from build123d import *

# Parameters (mm, degrees)
SKETCH1_W                     = 190.5
SKETCH1_H                     = 101.6
BOSS_EXTRUDE1_DEPTH           = 1.5875
CONVERT_SOLID1_START          = -95.25
CONVERT_SOLID1_OUTLINE_W      = 3.175
CONVERT_SOLID1_OUTLINE_H      = 101.6
CONVERT_SOLID1_DEPTH          = 190.5
SKETCH30_R                    = 12.770921212
CUT_EXTRUDE6_DEPTH            = 38.1
SKETCH35_W                    = 139.601875342
SKETCH35_H                    = 6.35
CUT_EXTRUDE7_DEPTH            = 0.254
EDGE_FLANGE1_STRIP_W          = 39.05
EDGE_FLANGE1_STRIP_H          = 4.7625
EDGE_FLANGE1_STRIP_CUT_DEPTH  = 25.449062329
EDGE_FLANGE1_RELIEF_W         = 41.43125
EDGE_FLANGE1_RELIEF_H         = 2.38125
EDGE_FLANGE1_RELIEF_CUT_DEPTH = 4.7625
EDGE_FLANGE1_DEPTH            = 25.449062329
EDGE_FLANGE2_STRIP_W          = 39.05
EDGE_FLANGE2_STRIP_H          = 4.7625
EDGE_FLANGE2_STRIP_CUT_DEPTH  = 25.449062329
EDGE_FLANGE2_RELIEF_W         = 41.43125
EDGE_FLANGE2_RELIEF_H         = 2.38125
EDGE_FLANGE2_RELIEF_CUT_DEPTH = 4.7625
EDGE_FLANGE2_DEPTH            = 25.449062329
SKETCH45_W                    = 4.7625
SKETCH45_H                    = 0.000254
CUT_EXTRUDE10_DEPTH           = 25.4
EDGE_FLANGE4_STRIP_W          = 39.05
EDGE_FLANGE4_STRIP_H          = 4.7625
EDGE_FLANGE4_STRIP_CUT_DEPTH  = 25.4
EDGE_FLANGE4_RELIEF_W         = 41.43125
EDGE_FLANGE4_RELIEF_H         = 2.38125
EDGE_FLANGE4_RELIEF_CUT_DEPTH = 4.7625
EDGE_FLANGE4_DEPTH            = 25.4
FILLET9_R                     = 25.4
CUT_EXTRUDE11_DEPTH           = 25.4
FILLET10_R                    = 25.4
SKETCH53_R                    = 2.54
CUT_EXTRUDE12_DEPTH           = 4.7625
SKETCH54_R                    = 2.54
CUT_EXTRUDE13_DEPTH           = 4.7625
SKETCH55_R                    = 9.525
SKETCH55_R_2                  = 2.54
CUT_EXTRUDE14_DEPTH           = 4.7625


# Read off the part's stored shape, not the designer's step: Convert-Solid1
# Sheet-metal steps are written as plain solids
with BuildPart() as part:
    # Sketch1 → Boss-Extrude1 (new body)
    with BuildSketch(Plane(origin=(0, 0, 0), x_dir=(1, 0, 0), z_dir=(0, 1, 0))):
        Rectangle(SKETCH1_W, SKETCH1_H)
    extrude(amount=BOSS_EXTRUDE1_DEPTH)

    # Convert-Solid1 outline → Convert-Solid1 (add)
    with BuildSketch(Plane.YZ.offset(CONVERT_SOLID1_START)):
        with Locations((-1.5875, 0)):
            Rectangle(CONVERT_SOLID1_OUTLINE_W, CONVERT_SOLID1_OUTLINE_H)
    extrude(amount=CONVERT_SOLID1_DEPTH)

    # Sketch30 → Cut-Extrude6 (cut)
    with BuildSketch(Plane(origin=(0, -3.175, 0), x_dir=(-1, 0, 0), z_dir=(0, -1, 0))):
        with Locations(Location((0, -25.504506424, 0), (0, 0, 90))):
            Circle(SKETCH30_R)
    extrude(amount=-CUT_EXTRUDE6_DEPTH, mode=Mode.SUBTRACT)

    # Sketch35 → Cut-Extrude7 (cut)
    with BuildSketch(Plane(origin=(0, 0, -50.8), x_dir=(-1, 0, 0), z_dir=(0, 0, -1))):
        Rectangle(SKETCH35_W, SKETCH35_H)
    extrude(amount=-CUT_EXTRUDE7_DEPTH, mode=Mode.SUBTRACT)

    # Edge-Flange1 strip (across the edge) → Edge-Flange1 strip cut (cut)
    with BuildSketch(Plane(origin=(95.25, 1.5875, -50.8), x_dir=(0, 0, 1), z_dir=(-1, 0, 0))):
        with Locations((-4.7625, -2.38125)):
            Rectangle(EDGE_FLANGE1_STRIP_W, EDGE_FLANGE1_STRIP_H)
    extrude(amount=EDGE_FLANGE1_STRIP_CUT_DEPTH, mode=Mode.SUBTRACT)

    # Edge-Flange1 relief (on the sheet) → Edge-Flange1 relief cut (cut)
    with BuildSketch(Plane(origin=(95.25, 1.5875, -36.0375), x_dir=(0, 0, 1), z_dir=(0, 1, 0))):
        with Locations((-18.334375, -26.639687329)):
            Rectangle(EDGE_FLANGE1_RELIEF_W, EDGE_FLANGE1_RELIEF_H)
    extrude(amount=-EDGE_FLANGE1_RELIEF_CUT_DEPTH, mode=Mode.SUBTRACT)

    # Edge-Flange1 section (across the edge) → Edge-Flange1 (add)
    with BuildSketch(Plane(origin=(95.25, 1.5875, -50.8), x_dir=(0, 0, 1), z_dir=(-1, 0, 0))):
        with BuildLine():
            Line((0, 10), (0, 46.0375))
            Line((0, 46.0375), (4.7625, 46.0375))
            Line((4.7625, 46.0375), (4.7625, 10))
            ThreePointArc((4.7625, 10), (7.691432188, 2.928932188), (14.7625, 0))
            Line((14.7625, 0), (14.7625, -4.7625))
            ThreePointArc((14.7625, -4.7625), (4.323836143, -0.438663857), (0, 10))
        make_face()
    extrude(amount=EDGE_FLANGE1_DEPTH)

    # Edge-Flange2 strip (across the edge) → Edge-Flange2 strip cut (cut)
    with BuildSketch(Plane(origin=(-69.800937671, 1.5875, -50.8), x_dir=(0, 0, 1), z_dir=(-1, 0, 0))):
        with Locations((-4.7625, -2.38125)):
            Rectangle(EDGE_FLANGE2_STRIP_W, EDGE_FLANGE2_STRIP_H)
    extrude(amount=EDGE_FLANGE2_STRIP_CUT_DEPTH, mode=Mode.SUBTRACT)

    # Edge-Flange2 relief (on the sheet) → Edge-Flange2 relief cut (cut)
    with BuildSketch(Plane(origin=(-69.800937671, 1.5875, -36.0375), x_dir=(0, 0, 1), z_dir=(0, 1, 0))):
        with Locations((-18.334375, 1.190625)):
            Rectangle(EDGE_FLANGE2_RELIEF_W, EDGE_FLANGE2_RELIEF_H)
    extrude(amount=-EDGE_FLANGE2_RELIEF_CUT_DEPTH, mode=Mode.SUBTRACT)

    # Edge-Flange2 section (across the edge) → Edge-Flange2 (add)
    with BuildSketch(Plane(origin=(-69.800937671, 1.5875, -50.8), x_dir=(0, 0, 1), z_dir=(-1, 0, 0))):
        with BuildLine():
            Line((0, 10), (0, 46.0375))
            Line((0, 46.0375), (4.7625, 46.0375))
            Line((4.7625, 46.0375), (4.7625, 10))
            ThreePointArc((4.7625, 10), (7.691432188, 2.928932188), (14.7625, 0))
            Line((14.7625, 0), (14.7625, -4.7625))
            ThreePointArc((14.7625, -4.7625), (4.323836143, -0.438663857), (0, 10))
        make_face()
    extrude(amount=EDGE_FLANGE2_DEPTH)

    # Sketch45 → Cut-Extrude10 (cut)
    with BuildSketch(Plane(origin=(0, 1.5875, 0), x_dir=(1, 0, 0), z_dir=(0, 1, 0))):
        with Locations((-92.86875, -25.399873)):
            Rectangle(SKETCH45_W, SKETCH45_H)
        with Locations((-92.86875, 0.000381)):
            Rectangle(SKETCH45_W, SKETCH45_H)
    extrude(amount=-CUT_EXTRUDE10_DEPTH, mode=Mode.SUBTRACT)

    # Edge-Flange4 strip (across the edge) → Edge-Flange4 strip cut (cut)
    with BuildSketch(Plane(origin=(-95.25, 1.5875, -0.000254), x_dir=(1, 0, 0), z_dir=(0, 0, 1))):
        with Locations((-9.525, -2.38125)):
            Rectangle(EDGE_FLANGE4_STRIP_W, EDGE_FLANGE4_STRIP_H)
    extrude(amount=EDGE_FLANGE4_STRIP_CUT_DEPTH, mode=Mode.SUBTRACT)

    # Edge-Flange4 relief (on the sheet) → Edge-Flange4 relief cut (cut)
    with BuildSketch(Plane(origin=(-85.25, 1.5875, -0.000254), x_dir=(1, 0, 0), z_dir=(0, 1, 0))):
        with Locations((-18.334375, 1.190625)):
            Rectangle(EDGE_FLANGE4_RELIEF_W, EDGE_FLANGE4_RELIEF_H)
        with Locations((-18.334375, -26.590625)):
            Rectangle(EDGE_FLANGE4_RELIEF_W, EDGE_FLANGE4_RELIEF_H)
    extrude(amount=-EDGE_FLANGE4_RELIEF_CUT_DEPTH, mode=Mode.SUBTRACT)

    # Edge-Flange4 section (across the edge) → Edge-Flange4 (add)
    with BuildSketch(Plane(origin=(-95.25, 1.5875, -0.000254), x_dir=(1, 0, 0), z_dir=(0, 0, 1))):
        with BuildLine():
            Line((-4.7625, 10), (-4.7625, 20.6375))
            Line((-4.7625, 20.6375), (0, 20.6375))
            Line((0, 20.6375), (0, 10))
            ThreePointArc((0, 10), (2.928932188, 2.928932188), (10, 0))
            Line((10, 0), (10, -4.7625))
            ThreePointArc((10, -4.7625), (-0.438663857, -0.438663857), (-4.7625, 10))
        make_face()
    extrude(amount=EDGE_FLANGE4_DEPTH)

    # Fillet9
    # the kernel refuses this fillet: 25.4 mm, written as the material it takes off along each edge
    with BuildSketch(Plane(origin=(-67.419687671, 61.417239936, -50.546), x_dir=(1, 0, 0), z_dir=(0, -1, 0))) as fillet9_piece_1:
        with BuildLine():
            CenterArc((23.931895975, 25.4), FILLET9_R, 199.575530564, 70.424469436)
            Line((0, 16.88975), (-0.478637919, 16.719545))
            ThreePointArc((-0.478637919, 16.719545), (-0.508, 8.444875), (-0.508, 0))
            Line((-0.508, 0), (0, -0.508))
            Line((0, -0.508), (23.931895975, -0.508))
            Line((23.931895975, -0.508), (23.931895975, 0))
        make_face()
    extrude(amount=124.421979873, mode=Mode.SUBTRACT)
    with BuildSketch(Plane(origin=(67.419687671, 61.417239936, -50.546), x_dir=(0, 0, 1), z_dir=(0, -1, 0))) as fillet9_piece_2:
        with BuildLine():
            CenterArc((25.4, 23.931895975), FILLET9_R, 180, 70.424469436)
            Line((0, 23.931895975), (-0.508, 23.931895975))
            Line((-0.508, 23.931895975), (-0.508, 0))
            Line((-0.508, 0), (0, -0.508))
            ThreePointArc((0, -0.508), (8.444875, -0.508), (16.719545, -0.478637919))
            Line((16.719545, -0.478637919), (16.88975, 0))
        make_face()
    extrude(amount=124.421979873, mode=Mode.SUBTRACT)

    # Sketch52 → Cut-Extrude11 (cut)
    with BuildSketch(Plane.XZ.offset(3.175)):
        with BuildLine():
            ThreePointArc((62.156767956, 50.8), (84.936935051, 40.486935051), (95.25, 17.706767956))
            Line((95.25, 17.706767956), (95.25, 50.8))
            Line((95.25, 50.8), (62.156767956, 50.8))
        make_face()
    extrude(amount=-CUT_EXTRUDE11_DEPTH, mode=Mode.SUBTRACT)

    # Fillet10
    # the kernel refuses this fillet: 25.4 mm, written as the material it takes off along each edge
    with BuildSketch(Plane(origin=(-95.25, 64.807891195, 50.8), x_dir=(1, 0, 0), z_dir=(0, -1, 0))) as fillet10_piece_1:
        with BuildLine():
            CenterArc((25.288156478, -25.4), FILLET10_R, 90, 84.621196501)
            Line((0, -23.019004), (-0.50576313, -22.97138408))
            ThreePointArc((-0.50576313, -22.97138408), (-0.508, -11.509502), (-0.508, 0))
            Line((-0.508, 0), (0, 0.508))
            Line((0, 0.508), (25.288156478, 0.508))
            Line((25.288156478, 0.508), (25.288156478, 0))
        make_face()
    extrude(amount=131.203282389, mode=Mode.SUBTRACT)

    # Sketch53 → Cut-Extrude12 (cut)
    with BuildSketch(Plane.ZY.offset(100.0125)):
        with Locations(Location((6.349746, 17.9375, 0), (0, 0, 270))):
            Circle(SKETCH53_R)
        with Locations(Location((19.049746, 17.9375, 0), (0, 0, 270))):
            Circle(SKETCH53_R)
    extrude(amount=-CUT_EXTRUDE12_DEPTH, mode=Mode.SUBTRACT)

    # Sketch54 → Cut-Extrude13 (cut)
    with BuildSketch(Plane(origin=(0, 0, -50.8), x_dir=(-1, 0, 0), z_dir=(0, 0, -1))):
        with Locations(Location((-82.55, 34.925, 0), (0, 0, 90))):
            Circle(SKETCH54_R)
        with Locations(Location((82.55, 34.925, 0), (0, 0, 90))):
            Circle(SKETCH54_R)
    extrude(amount=-CUT_EXTRUDE13_DEPTH, mode=Mode.SUBTRACT)

    # Sketch55 → Cut-Extrude14 (cut)
    with BuildSketch(Plane.XZ.offset(3.175)):
        with Locations(Location((-39.37, -21.037138368, 0), (0, 0, 270))):
            Circle(SKETCH55_R)
        with Locations(Location((39.37, -21.037138368, 0), (0, 0, 270))):
            Circle(SKETCH55_R)
        with Locations(Location((-17.001810213, -33.071426284, 0), (0, 0, 270))):
            Circle(SKETCH55_R_2)
        with Locations(Location((-61.002047674, -7.724944205, 0), (0, 0, 270))):
            Circle(SKETCH55_R_2)
        with Locations(Location((61.002047674, -7.724944205, 0), (0, 0, 270))):
            Circle(SKETCH55_R_2)
        with Locations(Location((17.001810213, -33.071426284, 0), (0, 0, 270))):
            Circle(SKETCH55_R_2)
    extrude(amount=-CUT_EXTRUDE14_DEPTH, mode=Mode.SUBTRACT)


solid = part.part
The listing builds one solid part. Answer for the finished solid, in the listing's coordinates (mm). A direction names the side the tool comes from. Give positions to 0.01 mm unless a question says otherwise; leave off trailing zeros. Loops run counter-clockwise (first coordinate to the right, second up) from the corner with the lowest first, then second, coordinate; pieces in that order, holes last. Notation, with made-up numbers: (18.5, 47) - (54.5, 47) arc R17 ccw to (54.5, 80) - close; hole circle Ø2 at (50, 73.5). An arc over 180 degrees is marked (long way). Answer as a JSON object with one key per item and string values.
1. Flat-ended cylindrical pins translate along their axes: pin 1 Ø12.5 at (x, y) = (-82.5, 21) entering from +Z; pin 2 Ø6 at (x, z) = (61, -7.72) entering from +Y; pin 3 Ø12 at (y, z) = (20.5, 1.5) entering from +X. Find the tip coordinate at first contact, or state that the pin passes through.
Determined:
{"pin 1": "z = -46.04", "pin 2": "y = 1.59", "pin 3": "x = -95.25"}
2. For a pull along X with two mould halves and no side action, classify faces 5 (the cylindrical face through (57.955, -0.76, -46.024)), 6 (the flat face through (-100.012, 17, 13)), 7 (the flat face through (-82, 30, -46.037)) as pulls with the +X half, pulls with the -X half, needs draft (parallel to the pull), parting line crosses it, or undercut.
Determined:
{"face 5": "undercut", "face 6": "pulls with the -X half", "face 7": "needs draft"}
3. A cutting plane is placed at A-A (y = 44). Write down the section's boundary in (x, z), then the cut area to 3 significant figures.
Determined:
{"outline": "(-95.25, -50.8) - (-69.8, -50.8) - (-69.8, -46.04) - (-95.25, -46.04) - close; (69.8, -50.8) - (95.25, -50.8) - (95.25, -46.04) - (69.8, -46.04) - close", "area": "242 mm²"}
4. A cutting plane is placed at C-C (z = -17). Give the number of separate pieces and of enclosed holes in the cut face, then the cut area to 3 significant figures.
Determined:
{"separate pieces": "3", "enclosed holes": "0", "area": "743 mm²"}
5. For faces 1 (the flat face through (83, 30, -46.037)), 2 (the cylindrical face through (-82.347, 4.595, -43.186)), 3 (the flat face through (-95.25, 14.8, -46.2)), 4 (the cylindrical face through (-92.398, 4.595, 12.522)), determine the directions among +Z, -Z, +X, -X, +Y, -Y from which every point of the face is accessible in a straight line to the end or side of a thin tool.
Determined:
{"face 1": "+Z, +X, -X, +Y", "face 2": "+X, -X, +Y", "face 3": "-Z, -X, +Y, -Y", "face 4": "+Z, +X, +Y"}
6. Find the intervals of material crossed by L1, parallel to Y at x = -30, z = 20 (1 decimal); L2, parallel to Z at x = -72.5, y = 24.5; L3, parallel to X at y = -0.5, z = 12, in increasing order. Write a range as [from, to].
Determined:
{"L1": "[-3.2, 1.6]", "L2": "[-50.8, -46.04]", "L3": "[-93.72, 95.25]"}
7. A cutting plane is placed at D-D (x = 82.55). Write down the section's boundary in (y, z) (1 decimal), then the cut area to 3 significant figures.
Determined:
{"outline": "(-3.2, -36) arc R14.8 ccw to (11.6, -50.8) - (32.4, -50.8) - (32.4, -46) - (11.6, -46) arc R10 cw to (1.6, -36) - (1.6, 42.7) - (-3.2, 42.7) - close; (37.5, -50.8) - (47.6, -50.8) - (47.6, -46) - (37.5, -46) - close", "area": "615 mm²"}
8. A cutting plane is placed at B-B (x = -39.37). Write down the section's boundary in (y, z) (1 decimal), then the cut area to 3 significant figures.
Determined:
{"outline": "(-3.2, -50.5) - (1.6, -50.5) - (1.6, -30.6) - (-3.2, -30.6) - close; (-3.2, -11.5) - (1.6, -11.5) - (1.6, 50.8) - (-3.2, 50.8) - close", "area": "392 mm²"}
